```python
from build123d import *

# Parameters (mm, degrees)
SKETCH1_W             = 128.922622712
SKETCH1_H             = 108.547542538
SKETCH1_W_2           = 124.922622712
SKETCH1_H_2           = 104.547542538
BOSS_EXTRUDE1_DEPTH   = 50
SKETCH2_R             = 48.496570744
BOSS_EXTRUDE2_DEPTH   = 50
SKETCH3_R             = 6.994110628
BOSS_EXTRUDE3_DEPTH   = 20
SKETCH3_R_2           = 6.120691225
BOSS_EXTRUDE3_2_DEPTH = 20


with BuildPart() as part:
    # Sketch1 → Boss-Extrude1 (new body)
    with BuildSketch(Plane.XY):
        Rectangle(SKETCH1_W, SKETCH1_H)
        Rectangle(SKETCH1_W_2, SKETCH1_H_2, mode=Mode.SUBTRACT)
    extrude(amount=BOSS_EXTRUDE1_DEPTH)


with BuildPart() as body_2:
    # Sketch2 → Boss-Extrude2 (new body)
    with BuildSketch(Plane.XY):
        with Locations(Location((0, 0, 0), (0, 0, 180))):
            Circle(SKETCH2_R)
    extrude(amount=BOSS_EXTRUDE2_DEPTH)


with BuildPart() as body_3:
    # Sketch3 → Boss-Extrude3 (new body)
    with BuildSketch(Plane.XY):
        with Locations((-51.126362865, 41.516845757)):
            Circle(SKETCH3_R)
    extrude(amount=BOSS_EXTRUDE3_DEPTH)


with BuildPart() as body_4:
    # Sketch3 → Boss-Extrude3 2 (new body)
    with BuildSketch(Plane.XY):
        with Locations((46.461548735, 43.755956539)):
            Circle(SKETCH3_R_2)
    extrude(amount=BOSS_EXTRUDE3_2_DEPTH)


solid = part.part
```
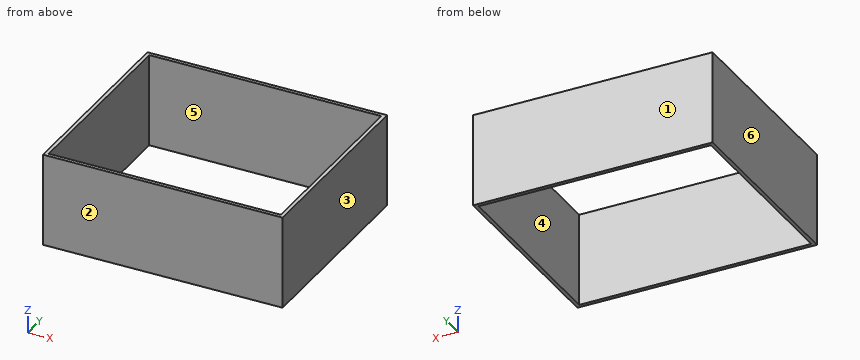
Work out the finished part from the listing and answer in its coordinate system (mm). Face numbers are marked on the shaded views. A direction names the side the tool comes from. Coordinates: 2 decimals unless noted, no trailing zeros. Write each loop counter-clockwise with the first axis right and the second up, starting at its lowest first coordinate (ties: lowest second). Pieces come first, ordered by that corner, then holes. Notation, with made-up numbers: (81.25, 13) - (101.25, 13) arc R28 cw to (101.25, 50) - close; hole circle Ø4 at (55, 71). An arc over 180 degrees is marked (long way). Answer as a JSON object with one key per item and string values.
Q1. Find section B-B (x = 25.5). Write down the section's boundary in (y, z), plus the area to 3 significant figures.
Results list:
{"outline": "(-54.27, 0) - (-52.27, 0) - (-52.27, 50) - (-54.27, 50) - close; (52.27, 0) - (54.27, 0) - (54.27, 50) - (52.27, 50) - close", "area": "200 mm^2"}
Q2. For a pull along Y with two mould halves and no side action, classify the marked faces 1, 2, 3 and 4 as pulls with the +Y half, pulls with the -Y half, needs draft (parallel to the pull), parting line crosses it, or undercut.
Results list:
{"face 1": "pulls with the +Y half", "face 2": "pulls with the -Y half", "face 3": "needs draft", "face 4": "undercut"}
Q3. Find section C-C (z = 28.5). Write down the section's boundary in (x, y).
Results list:
{"outline": "(-64.46, -54.27) - (64.46, -54.27) - (64.46, 54.27) - (-64.46, 54.27) - close; hole (-62.46, -52.27) - (62.46, -52.27) - (62.46, 52.27) - (-62.46, 52.27) - close"}
Q4. Which of the six approach directions +Z, -Z, +X, -X, +Y, -Y give full straight-line access (tool end or side, diameter ignored) to the marked faces 5 and 6?
Results list:
{"face 5": "+Z, -Z", "face 6": "+Z, -Z, -X, +Y, -Y"}
Q5. Find section A-A (y = 10). Write down the section's boundary in (x, z).
Results list:
{"outline": "(-64.46, 0) - (-62.46, 0) - (-62.46, 50) - (-64.46, 50) - close; (62.46, 0) - (64.46, 0) - (64.46, 50) - (62.46, 50) - close"}
Q6. Consider L1, parallel to Y at x = -19, z = 42; L2, parallel to X at y = -30, z = 17. Determine where each line is inside the solid, lowest interval first. Write a range as from..to.
Results list:
{"L1": "y = -54.27..-52.27, 52.27..54.27", "L2": "x = -64.46..-62.46, 62.46..64.46"}
